from build123d import *

# Parameters (mm, degrees)
F0_R     = 5
F0_R_2   = 2.25
F1_DEPTH = 5


# Not quite as in the source:
# - a fillet or chamfer that OpenCascade refuses, or shapes differently, is made with other operations: its cross-section is extruded or revolved along the edge and cut away or added


with BuildPart() as f1:
    # F0 (on Front) → F1 (new body)
    with BuildSketch(Plane.XZ):
        with BuildLine():
            Line((54.5685509182, 10), (-38.6314490818, 10))
            ThreePointArc((-38.6314490818, 10), (-47.6314490818, 1), (-38.6314490818, -8))
            Line((-38.6314490818, -8), (54.5685509182, -8))
            Line((54.5685509182, -8), (54.5685509182, 10))
        make_face()
        with Locations((-38.6314490818, 0)):
            Circle(F0_R, mode=Mode.SUBTRACT)
        with BuildLine():
            ThreePointArc((-22.6314490818, -4.25), (-26.8814490818, 0), (-22.6314490818, 4.25))
            Line((-22.6314490818, 4.25), (29.5685509182, 4.25))
            ThreePointArc((29.5685509182, 4.25), (33.8185509182, 0), (29.5685509182, -4.25))
            Line((29.5685509182, -4.25), (-22.6314490818, -4.25))
        make_face(mode=Mode.SUBTRACT)
        with Locations((49.5685509182, 0)):
            Circle(F0_R_2, mode=Mode.SUBTRACT)
        with Locations((-15.4314490818, 7.5)):
            Circle(F0_R_2, mode=Mode.SUBTRACT)
        with Locations((19.5685509182, 7.5)):
            Circle(F0_R_2, mode=Mode.SUBTRACT)
    extrude(amount=F1_DEPTH)

    # F2: chamfer of 1 on 3 edges, made by hand

    # F2_s1 → F2_t2 (revolve, cut)
    with BuildSketch(Plane.XY.offset(7.5)):
        Polygon((-13.1814490818, -4), (-12.1814490818, -5), (-13.1814490818, -5), align=None)
    revolve(axis=Axis((-15.4314490818, -5, 7.5), (0, -1, 0)), mode=Mode.SUBTRACT)

    # F2_s3 → F2_t4 (revolve, cut)
    with BuildSketch(Plane.XY.offset(7.5)):
        Polygon((21.8185509182, -4), (22.8185509182, -5), (21.8185509182, -5), align=None)
    revolve(axis=Axis((19.5685509182, -5, 7.5), (0, -1, 0)), mode=Mode.SUBTRACT)

    # F2_s5 → F2_t6 (revolve, cut)
    with BuildSketch(Plane.XY):
        Polygon((51.8185509182, -4), (52.8185509182, -5), (51.8185509182, -5), align=None)
    revolve(axis=Axis((49.5685509182, -5, 0), (0, -1, 0)), mode=Mode.SUBTRACT)


solid = f1.part
Check sheet for the modelled part. Datum: model origin and axes. Units: mm. A direction names the side the tool comes from. Coordinates: 2 decimals unless noted, no trailing zeros. Write each loop counter-clockwise with the first axis right and the second up, starting at its lowest first coordinate (ties: lowest second). Pieces come first, ordered by that corner, then holes.
Item 1: Cross-section at A-A on x = 12.5. Record the boundary of the cut face in (y, z).
Numbers:
outline: (-5, -8) - (0, -8) - (0, -4.25) - (-5, -4.25) - close; (-5, 4.25) - (0, 4.25) - (0, 10) - (-5, 10) - close
Item 2: Access from +Z, -Z, +X, -X, +Y, -Y to the whole of each face (thin tool, end or side, straight path). Record for faces 1 (the face through (9, -2, 10)), 2 (the face through (-26.88, -2.46, -0.09)).
Numbers:
face 1: +Z, +X, -X, +Y, -Y
face 2: +Y, -Y
Item 3: Depth check by flat-ended pin: pin 1 Ø1 at (y, z) = (-2.5, 5) entering from -X; pin 2 Ø6 at (x, z) = (36.5, -3) entering from +Y. Enter the tip coordinate at first touch or a pass-through.
Numbers:
pin 1: stops at x = -46.92
pin 2: stops at y = 0
Item 4: Cross-section at B-B on z = 0. Record the boundary of the cut face in (x, y).
Numbers:
outline: (-47.58, -5) - (-43.63, -5) - (-43.63, 0) - (-47.58, 0) - close; (-33.63, -5) - (-26.88, -5) - (-26.88, 0) - (-33.63, 0) - close; (33.82, -5) - (46.32, -5) - (47.32, -4) - (47.32, 0) - (33.82, 0) - close; (51.82, -4) - (52.82, -5) - (54.57, -5) - (54.57, 0) - (51.82, 0) - close
Item 5: Cross-section at D-D on z = 7.5. Record the boundary of the cut face in (x, y).
Numbers:
outline: (-44.86, -5) - (-18.68, -5) - (-17.68, -4) - (-17.68, 0) - (-44.86, 0) - close; (-13.18, -4) - (-12.18, -5) - (16.32, -5) - (17.32, -4) - (17.32, 0) - (-13.18, 0) - close; (21.82, -4) - (22.82, -5) - (54.57, -5) - (54.57, 0) - (21.82, 0) - close
Item 6: Cross-section at C-C on y = -3.15. Record the boundary of the cut face in (x, z), then the cut area to 3 significant figures.
Numbers:
outline: (-38.63, -8) - (54.57, -8) - (54.57, 10) - (-38.63, 10) arc R9 ccw to start; hole circle Ø10 at (-38.63, 0); hole (-22.63, -4.25) - (29.57, -4.25) arc R4.25 ccw to (29.57, 4.25) - (-22.63, 4.25) arc R4.25 ccw to start; hole circle Ø4.5 at (-15.43, 7.5); hole circle Ø4.5 at (19.57, 7.5); hole circle Ø4.5 at (49.57, 0)
area: 1,180 mm2
Item 7: Mould release check, pull along X, two halves, no side actions. Record for faces 3 (the face through (21.715, -1.972, 8.176)), 4 (the face through (3, -5, -5)), 5 (the face through (-47.63, -2.46, 1.2)), 6 (the face through (19.043, -4.174, 5.134)): released by +X, released by -X, zero draft, split by the parting line, or undercut.
Numbers:
face 3: undercut
face 4: zero draft
face 5: released by -X
face 6: undercut
Item 8: Scan lines: probe 1 along Z at (x, y) = (19.5, -3.1); probe 2 along Z at (x, y) = (-21, -4.45); probe 3 along Z at (x, y) = (-13, -4.7). Record each from-to range of solid material in increasing order.
Numbers:
probe 1: z = -8 to -4.25, 4.25 to 5.25, 9.75 to 10
probe 2: z = -8 to -4.25, 4.25 to 10
probe 3: z = -8 to -4.25, 4.25 to 5.83, 9.17 to 10
